Job drawing, mm, ordinate dimensions from the low corner. One solid piece. A direction names the side the tool comes from. Coordinates: 2 decimals unless noted, no trailing zeros. Order: outer loops, then holes, each group sorted by start corner. A loop starts at its lowest first (then second) coordinate and runs counter-clockwise, first axis right, second up. Notation, with made-up numbers: (73.5, -35) - (87.5, -35) arc R14 cw to (87.5, -17) - close; hole circle Ø5 at (49, -37.75). An arc over 180 degrees is marked (long way). Return JSON: item names as keys, results as strings.
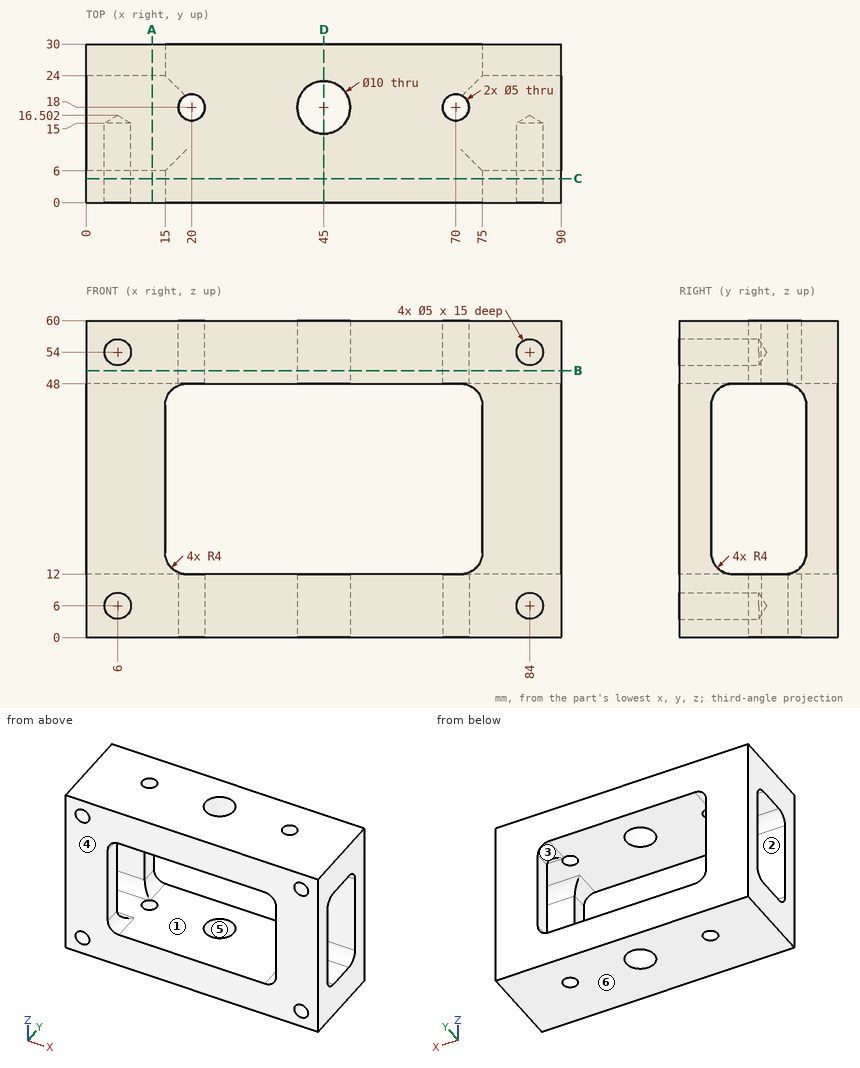
1. Cut at C-C on y = 4.5. Give the cut face in (x, z).
Check values:
{"outline": "(0, 0) - (90, 0) - (90, 60) - (0, 60) - close; hole circle Ø5 at (6, 6); hole circle Ø5 at (6, 54); hole (15, 16) arc R4 ccw to (19, 12) - (71, 12) arc R4 ccw to (75, 16) - (75, 44) arc R4 ccw to (71, 48) - (19, 48) arc R4 ccw to (15, 44) - close; hole circle Ø5 at (84, 6); hole circle Ø5 at (84, 54)"}
2. Drop flat-ended pins along their axis: pin 1 (3 mm diameter, centred on x = 70, y = 18, fed in from -Z); pin 2 (4 mm diameter, centred on x = 84, z = 54, fed in from -Y); pin 3 (4.5 mm diameter, centred on x = 6, z = 6, fed in from -Y); pin 4 (3 mm diameter, centred on x = 84, z = 6, fed in from -Y). Give the stop position or say it passes through.
Check values:
{"pin 1": "through", "pin 2": "y = 15.3", "pin 3": "y = 15.15", "pin 4": "y = 15.6"}
3. Mould opens along Y. For the marked faces 4, 5 and 6 say: pulls with the +Y half, pulls with the -Y half, needs draft (parallel to the pull), parting line crosses it, or undercut.
Check values:
{"face 4": "pulls with the -Y half", "face 5": "undercut", "face 6": "needs draft"}
4. Cut at B-B on z = 50.5. Give the cut face in (x, y), plus the area to 3 significant figures.
Check values:
{"outline": "(0, 0) - (90, 0) - (90, 30) - (0, 30) - close; hole circle Ø5 at (20, 18); hole circle Ø10 at (45, 18); hole circle Ø5 at (70, 18)", "area": "2,580 mm²"}
5. Probe L1, parallel to Z at x = 51, y = 18; L2, parallel to X at y = 2, z = 18; L3, parallel to X at y = 18, z = 56. List the from-to ranges inside material, lowest first.
Check values:
{"L1": "0 to 12, 48 to 60", "L2": "0 to 15, 75 to 90", "L3": "0 to 17.5, 22.5 to 40, 50 to 67.5, 72.5 to 90"}
6. Tool access for the marked faces 1, 2 and 3: list every direction of +Z, -Z, +X, -X, +Y, -Y with a clear straight run to the whole face (end or side of a thin tool).
Check values:
{"face 1": "none", "face 2": "+X, -X", "face 3": "+Y, -Y"}
7. Cut at A-A on x = 12.5. Give the cut face in (y, z), plus the area to 3 significant figures.
Check values:
{"outline": "(0, 0) - (30, 0) - (30, 60) - (0, 60) - close; hole (6, 16) arc R4 ccw to (10, 12) - (20, 12) arc R4 ccw to (24, 16) - (24, 44) arc R4 ccw to (20, 48) - (10, 48) arc R4 ccw to (6, 44) - close", "area": "1,170 mm²"}
8. Cut at D-D on x = 45. Give the cut face in (y, z).
Check values:
{"outline": "(0, 0) - (13, 0) - (13, 12) - (0, 12) - close; (0, 48) - (13, 48) - (13, 60) - (0, 60) - close; (23, 0) - (30, 0) - (30, 12) - (23, 12) - close; (23, 48) - (30, 48) - (30, 60) - (23, 60) - close"}
